from build123d import *

# Parameters (mm, degrees)
SKETCH1_W                                    = 30
SKETCH1_H                                    = 30
SKETCH1_R                                    = 10
BOSS_EXTRUDE1_DEPTH                          = 40
CUT_EXTRUDE1_DEPTH                           = 59.309518948
CUT_EXTRUDE2_DEPTH                           = 59.309518948
BOSS_EXTRUDE2_DEPTH                          = 40
FILLET1_R                                    = 6
M3_CLEARANCE_HOLE1_D                         = 3.2
M3_CLEARANCE_HOLE1_CSINK_D                   = 3.25
M3_CLEARANCE_HOLE1_CSINK_ANGLE               = 90
CBORE_FOR_M3_HEX_SOCKET_HEAD_CAP_SCR_2_COUNT = 2
CBORE_FOR_M3_HEX_SOCKET_HEAD_CAP_SCR_2_PITCH = 12
CBORE_FOR_M3_HEX_SOCKET_HEAD_CAP_SCR_3_COUNT = 2
CBORE_FOR_M3_HEX_SOCKET_HEAD_CAP_SCR_3_PITCH = 24
CBORE_FOR_M3_HEX_SOCKET_HEAD_CAP_SCR_4_COUNT = 2
CBORE_FOR_M3_HEX_SOCKET_HEAD_CAP_SCR_4_PITCH = 30.426406871
CBORE_FOR_M3_HEX_SOCKET_HEAD_CAP_SCR_5_COUNT = 2
CBORE_FOR_M3_HEX_SOCKET_HEAD_CAP_SCR_5_PITCH = 32.707281072
CBORE_FOR_M3_HEX_SOCKET_HEAD_CAP_SCR_6_COUNT = 2
CBORE_FOR_M3_HEX_SOCKET_HEAD_CAP_SCR_6_PITCH = 38.752628751
SKETCH10_R                                   = 3.25
CUT_EXTRUDE3_DEPTH                           = 47.55178469
FILLET2_R                                    = 10


with BuildPart() as part:
    # Sketch1 → Boss-Extrude1 (new body)
    with BuildSketch(Plane(origin=(0, 0, 0), x_dir=(1, 0, 0), z_dir=(0, 1, 0))):
        with Locations((15, 15)):
            Rectangle(SKETCH1_W, SKETCH1_H)
        with Locations(Location((15, 15, 0), (0, 0, 270))):
            Circle(SKETCH1_R, mode=Mode.SUBTRACT)
    extrude(amount=BOSS_EXTRUDE1_DEPTH)

    # Sketch2 → Cut-Extrude1 (cut, through all)
    with BuildSketch(Plane(origin=(0, 40, 0), x_dir=(1, 0, 0), z_dir=(0, 1, 0))):
        with BuildLine():
            Line((5, 15), (5, 30))
            Line((5, 30), (30, 30))
            Line((30, 30), (30, 5))
            Line((30, 5), (15, 5))
            ThreePointArc((15, 5), (7.928932188, 7.928932188), (5, 15))
        make_face()
    extrude(amount=-CUT_EXTRUDE1_DEPTH, mode=Mode.SUBTRACT)

    # Sketch3 → Cut-Extrude2 (cut, through all)
    with BuildSketch(Plane(origin=(0, 40, 0), x_dir=(1, 0, 0), z_dir=(0, 1, 0))):
        Polygon((0, 30), (5, 25), (5, 30), align=None)
        Polygon((30, 0), (25, 5), (30, 5), align=None)
    extrude(amount=-CUT_EXTRUDE2_DEPTH, mode=Mode.SUBTRACT)

    # Sketch7 → Boss-Extrude2 (add)
    with BuildSketch(Plane(origin=(0, 40, 0), x_dir=(1, 0, 0), z_dir=(0, 1, 0))):
        Polygon((5, 25), (8, 22), (5, 22), align=None)
        Polygon((25, 5), (22, 8), (22, 5), align=None)
    extrude(amount=-BOSS_EXTRUDE2_DEPTH)

    # Fillet1
    # the kernel refuses this fillet: 6 mm, written as the material it adds along each edge
    with BuildSketch(Plane(origin=(5, 40, -22), x_dir=(1, 0, 0), z_dir=(0, -1, 0))) as fillet1_piece_1_section:
        with BuildLine():
            CenterArc((6, 5.196152423), FILLET1_R, 180, 60)
            Line((0, 5.196152423), (-0.12, 5.196152423))
            Line((-0.12, 5.196152423), (-0.12, 0))
            Line((-0.12, 0), (0, -0.12))
            ThreePointArc((0, -0.12), (1.5, -0.12), (2.94, -0.103923048))
            Line((2.94, -0.103923048), (3, 0))
        make_face()
    fillet1_piece_1 = extrude(amount=40, mode=Mode.PRIVATE)
    fillet1_piece_1 = split(fillet1_piece_1, bisect_by=Plane(origin=(7.537314478, 20, -22.462685522), z_dir=(-0.7071067811865479, 0, 0.7071067811865474)), keep=Keep.TOP, mode=Mode.PRIVATE)
    add(fillet1_piece_1)
    with BuildSketch(Plane(origin=(22, 40, -5), x_dir=(-1, 0, 0), z_dir=(0, -1, 0))) as fillet1_piece_2_section:
        with BuildLine():
            CenterArc((5.196152423, 6), FILLET1_R, 210, 60)
            Line((0, 3), (-0.103923048, 2.94))
            ThreePointArc((-0.103923048, 2.94), (-0.12, 1.5), (-0.12, 0))
            Line((-0.12, 0), (0, -0.12))
            Line((0, -0.12), (5.196152423, -0.12))
            Line((5.196152423, -0.12), (5.196152423, 0))
        make_face()
    fillet1_piece_2 = extrude(amount=40, mode=Mode.PRIVATE)
    fillet1_piece_2 = split(fillet1_piece_2, bisect_by=Plane(origin=(22.462685522, 20, -7.537314478), z_dir=(-0.7071067811865436, 0, 0.7071067811865516)), keep=Keep.TOP, mode=Mode.PRIVATE)
    add(fillet1_piece_2)

    # M3 Clearance Hole1 (through all)
    with Locations(Plane(origin=(15, 0, -15), x_dir=(-0.7071067811865475, 0, -0.7071067811865476), z_dir=(0.7071067811865476, 0, -0.7071067811865475))):
        with Locations((-15.213203436, 32), (15.213203436, 32), (15.213203436, 20), (15.213203436, 8), (-15.213203436, 8), (-15.213203436, 20)):
            CounterSinkHole(M3_CLEARANCE_HOLE1_D / 2, M3_CLEARANCE_HOLE1_CSINK_D / 2, counter_sink_angle=M3_CLEARANCE_HOLE1_CSINK_ANGLE)

    # Sketch9 → CBORE for M3 Hex Socket Head Cap Screw1 (revolve, cut)
    with BuildSketch(Plane(origin=(21.514718626, 32, 0), x_dir=(0.7071067811865515, 0, 0.7071067811865436), z_dir=(0, 1, 0))):
        Polygon((0, 0), (0, 27.213203436), (1.7, 27.213203436), (1.7, 3.4), (3.25, 3.4), (3.25, 0.025), (3.275, 0), align=None)
    cbore_for_m3_hex_socket_head_cap_screw1 = revolve(axis=Axis((17.024590565, 32, 4.490128061), (0.7071067811865436, 0, -0.7071067811865515)), mode=Mode.SUBTRACT)

    # CBORE for M3 Hex Socket Head Cap Scr 2: CBORE for M3 Hex Socket Head Cap Screw1 ×2
    with Locations(*[(0, -i * CBORE_FOR_M3_HEX_SOCKET_HEAD_CAP_SCR_2_PITCH, 0) for i in range(1, CBORE_FOR_M3_HEX_SOCKET_HEAD_CAP_SCR_2_COUNT)]):
        add(cbore_for_m3_hex_socket_head_cap_screw1, mode=Mode.SUBTRACT)

    # CBORE for M3 Hex Socket Head Cap Scr 3: CBORE for M3 Hex Socket Head Cap Screw1 ×2
    with Locations(*[(0, -i * CBORE_FOR_M3_HEX_SOCKET_HEAD_CAP_SCR_3_PITCH, 0) for i in range(1, CBORE_FOR_M3_HEX_SOCKET_HEAD_CAP_SCR_3_COUNT)]):
        add(cbore_for_m3_hex_socket_head_cap_screw1, mode=Mode.SUBTRACT)

    # CBORE for M3 Hex Socket Head Cap Scr 4: CBORE for M3 Hex Socket Head Cap Screw1 ×2
    with Locations(*[Vector(-0.7071067811865515, 0, -0.7071067811865437) * (i * CBORE_FOR_M3_HEX_SOCKET_HEAD_CAP_SCR_4_PITCH) for i in range(1, CBORE_FOR_M3_HEX_SOCKET_HEAD_CAP_SCR_4_COUNT)]):
        add(cbore_for_m3_hex_socket_head_cap_screw1, mode=Mode.SUBTRACT)

    # CBORE for M3 Hex Socket Head Cap Scr 5: CBORE for M3 Hex Socket Head Cap Screw1 ×2
    with Locations(*[Vector(-0.6577959989617107, -0.3668907841578198, -0.6577959989617034) * (i * CBORE_FOR_M3_HEX_SOCKET_HEAD_CAP_SCR_5_PITCH) for i in range(1, CBORE_FOR_M3_HEX_SOCKET_HEAD_CAP_SCR_5_COUNT)]):
        add(cbore_for_m3_hex_socket_head_cap_screw1, mode=Mode.SUBTRACT)

    # CBORE for M3 Hex Socket Head Cap Scr 6: CBORE for M3 Hex Socket Head Cap Screw1 ×2
    with Locations(*[Vector(-0.5551808824158828, -0.6193128253151639, -0.5551808824158766) * (i * CBORE_FOR_M3_HEX_SOCKET_HEAD_CAP_SCR_6_PITCH) for i in range(1, CBORE_FOR_M3_HEX_SOCKET_HEAD_CAP_SCR_6_COUNT)]):
        add(cbore_for_m3_hex_socket_head_cap_screw1, mode=Mode.SUBTRACT)

    # Sketch10 → Cut-Extrude3 (cut, through all)
    with BuildSketch(Plane(origin=(13.161522369, 0, -13.161522369), x_dir=(0.7071067811865515, 0, 0.7071067811865436), z_dir=(-0.7071067811865436, 0, 0.7071067811865515))):
        with Locations((-15.213203436, 8)):
            Circle(SKETCH10_R)
        with Locations((-15.213203436, 20)):
            Circle(SKETCH10_R)
        with Locations((-15.213203436, 32)):
            Circle(SKETCH10_R)
        with Locations((15.213203436, 32)):
            Circle(SKETCH10_R)
        with Locations((15.213203436, 20)):
            Circle(SKETCH10_R)
        with Locations((15.213203436, 8)):
            Circle(SKETCH10_R)
    extrude(amount=CUT_EXTRUDE3_DEPTH, mode=Mode.SUBTRACT)

    # Fillet2
    fillet2_edges = [part.edges().sort_by_distance(p)[0] for p in [
        (0, 20, 0),
    ]]
    fillet(fillet2_edges, radius=FILLET2_R)


solid = part.part
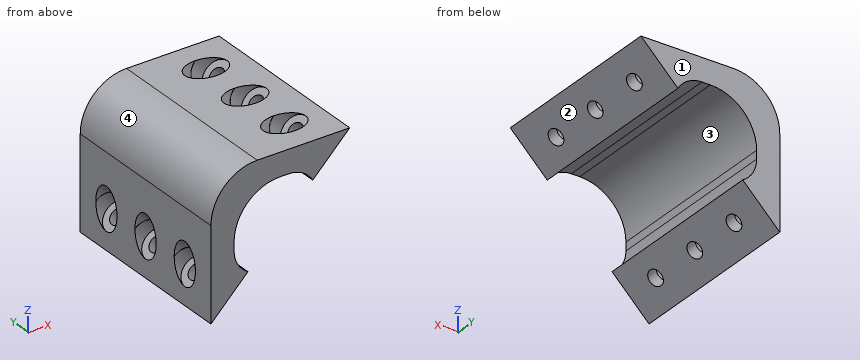
Work out the finished part from the listing and answer in its coordinate system (mm). Face numbers are marked on the shaded views. Coordinates: 2 decimals unless noted, no trailing zeros. Loops run counter-clockwise (first coordinate to the right, second up) from the corner with the lowest first, then second, coordinate; pieces in that order, holes last. Notation, with made-up numbers: M -16.75,45.5 L 16.25,45.5 A10 ccw 16.25,61.5 Z; hole C -13.5,47.5 d4. An arc over 180 degrees is marked long. Answer in a Markdown table with one row per item. Add a question column.
1. Find section A-A, the plane y = 12.5. Write down the section's boundary in (x, z).
2. Flat-ended cylindrical pins translate along their axes: P1, Ø6, axis at x = 21.5, y = 11.5, coming from the -Z side; P2, Ø0.9, axis at y = 26, z = -16, coming from the +X side; P3, Ø0.5, axis at x = 16, y = 15.5, coming from the -Z side; P4, Ø5, axis at x = 12.5, z = -8.5, coming from the +Y side. Find the tip coordinate at first contact, or state that the pin passes through.
3. The mould has two halves that part along Z. Classify the marked faces 1, 2, 3 and 4: pulls with the +Z half, pulls with the -Z half, needs draft (parallel to the pull), parting line crosses it, or undercut.
4. Find section C-C, the plane x = 6.5. Write down the section's boundary in (y, z), then the cut area to 3 significant figures.
5. Find section D-D, the plane z = -16.25. Write down the section's boundary in (x, y), then the cut area to 3 significant figures.
6. Find section B-B, the plane z = -7.5. Write down the section's boundary in (x, y), then the cut area to 3 significant figures.
7. Consider L1, parallel to Z at x = 16.5, y = 9; L2, parallel to X at y = 24.5, z = -6; L3, parallel to X at y = 23, z = -7.25. Determine where each line is inside the solid, lowest interval first.
Reported:
| question | item | result |
|---|---|---|
| 1 | outline | M 0,-30 L 8,-22 A6 cw 5,-16.8 L 5,-15 A10 cw 15,-5 L 16.8,-5 A6 cw 22,-8 L 30,0 L 10,0 A10 ccw 0,-10 Z |
| 2 | P1 | stops at z = -8 |
| 2 | P2 | stops at x = 5 |
| 2 | P3 | stops at z = -5 |
| 2 | P4 | passes through |
| 3 | face 1 | needs draft |
| 3 | face 2 | pulls with the -Z half |
| 3 | face 3 | undercut |
| 3 | face 4 | pulls with the +Z half |
| 4 | outline | M 0,-23.5 L 40,-23.5 L 40,-20.77 L 0,-20.77 Z; M 0,-9.73 L 40,-9.73 L 40,-0.63 L 0,-0.63 Z |
| 4 | area | 473 mm^2 |
| 5 | outline | M 0,0 L 5,0 L 5,40 L 0,40 Z |
| 5 | area | 200 mm^2 |
| 6 | outline | M 0.32,0 L 8.39,0 L 8.39,40 L 0.32,40 Z; M 21.68,0 L 22.5,0 L 22.5,40 L 21.68,40 Z |
| 6 | area | 356 mm^2 |
| 7 | L1 | z = -5 to 0 |
| 7 | L2 | x = 0.83 to 10.64, 20.12 to 24 |
| 7 | L3 | x = 0.39 to 8.68, 21.49 to 22.75 |
